from build123d import *

# Parameters (mm, degrees)
F0_W     = 26
F0_H     = 46
F1_DEPTH = 26
F2_W     = 10
F2_H     = 10
F3_DEPTH = 11
F4_W     = 10
F4_H     = 10
F5_DEPTH = 11
F7_R     = 1.55
F8_DEPTH = 26
F6_R     = 11
F9_DEPTH = 26


with BuildPart() as f1:
    # F0 (on Front) → F1 (new body)
    with BuildSketch(Plane.XZ):
        with Locations((13, 23)):
            Rectangle(F0_W, F0_H)
    extrude(amount=F1_DEPTH)

    # F2 (on face) → F3 (cut)
    with BuildSketch(Plane.XY.offset(46)):
        with Locations((13, -13)):
            Rectangle(F2_W, F2_H)
    extrude(amount=-F3_DEPTH, mode=Mode.SUBTRACT)

    # F4 (on face) → F5 (cut)
    with BuildSketch(Plane(origin=(0, 0, 0), x_dir=(1, 0, 0), z_dir=(0, 0, -1))):
        with Locations((13, 13)):
            Rectangle(F4_W, F4_H)
    extrude(amount=-F5_DEPTH, mode=Mode.SUBTRACT)

    # F7 (on face) → F8 (cut)
    with BuildSketch(Plane(origin=(0, 0, 0), x_dir=(0, -1, 0), z_dir=(-1, 0, 0))):
        with Locations((13, 8.5)):
            Circle(F7_R)
        with Locations((13, 3.5)):
            Circle(F7_R)
        with Locations((13, 42.5)):
            Circle(F7_R)
        with Locations((13, 37.5)):
            Circle(F7_R)
    extrude(amount=-F8_DEPTH, mode=Mode.SUBTRACT)

    # F6 (on face) → F9 (cut)
    with BuildSketch(Plane.YZ.offset(26)):
        with Locations((-13, 23)):
            Circle(F6_R)
    extrude(amount=-F9_DEPTH, mode=Mode.SUBTRACT)


solid = f1.part
Build history of the part. All positions in model axes, mm. A direction names the side the tool comes from. Give positions to 0.01 mm unless a question says otherwise; leave off trailing zeros. Order: outer loops, then holes, each group sorted by start corner. A loop starts at its lowest first (then second) coordinate and runs counter-clockwise, first axis right, second up. Notation, with made-up numbers: M 49,10.25 L 107,10.25 A20 cw 107,35.25 Z; hole C -35,58.25 d8. An arc over 180 degrees is marked long. Put each result on its own line as item: value.
Item 1: Slice it at D-D, the plane y = -7.5. Write the cut outline in (x, z), plus the area to 3 significant figures.
From the geometry:
outline: M 0,0 L 26,0 L 26,13.47 L 0,13.47 Z; M 0,32.53 L 26,32.53 L 26,46 L 0,46 Z
area: 701 mm2
Item 2: Two-plate mould, pull along Z, no slides. Class faces 4 (the cylindrical face through (13.18, -15.38, 12.26)), 5 (the cylindrical face through (3.944, -12.664, 40.987)), 6 (the flat face through (13, -13, 35)), 7 (the flat face through (8, -12.9, 5.4)): +Z half, -Z half, draft (parallel to the pull), parting line (faces both ways), or undercut.
From the geometry:
face 4: undercut
face 5: undercut
face 6: +Z half
face 7: draft
Item 3: Probe line 1 (Z direction, x = 3, y = -13); line 2 (X direction, y = -16.5, z = 10); line 3 (Z direction, x = 19.75, y = -20). List the from-to ranges inside material, lowest first. Write a range as [from, to].
From the geometry:
line 1: z = [0, 1.95], [5.05, 6.95], [10.05, 12], [34, 35.95], [39.05, 40.95], [44.05, 46]
line 2: x = [0, 8], [18, 26]
line 3: z = [0, 14.51], [31.49, 46]
Item 4: 3-axis set-ups, long thin cutter, end or side, ignore diameter. For faces 1 (the flat face through (8, -13.1, 40.6)), 2 (the flat face through (18, -12.9, 5.4)), 3 (the cylindrical face through (3.944, -12.664, 35.987)): which of +Z, -Z, +X, -X, +Y, -Y reach the whole face in a straight line?
From the geometry:
face 1: +Z
face 2: -Z
face 3: +X, -X
Item 5: Slice it at A-A, the plane z = 23. Write the cut outline in (x, y), plus the area to 3 significant figures.
From the geometry:
outline: M 0,-26 L 26,-26 L 26,-24 L 0,-24 Z; M 0,-2 L 26,-2 L 26,0 L 0,0 Z
area: 104 mm2
Item 6: Slice it at C-C, the plane x = 4. Write the cut outline in (y, z), plus the area to 3 significant figures.
From the geometry:
outline: M -26,0 L 0,0 L 0,46 L -26,46 Z; hole C -13,23 d22; hole C -13,3.5 d3.1; hole C -13,8.5 d3.1; hole C -13,37.5 d3.1; hole C -13,42.5 d3.1
area: 786 mm2
Item 7: Slice it at B-B, the plane x = 12. Write the cut outline in (y, z), plus the area to 3 significant figures.
From the geometry:
outline: M -26,0 L -18,0 L -18,11 L -8,11 L -8,0 L 0,0 L 0,46 L -8,46 L -8,35 L -18,35 L -18,46 L -26,46 Z; hole C -13,23 d22
area: 596 mm2
Item 8: Flat gauge pins, fed straight in: pin 1 Ø10 at (x, y) = (17, -20.5) entering from -Z; pin 2 Ø10 at (y, z) = (-12, 25) entering from +X. Where does each tip first touch, or does it go through?
From the geometry:
pin 1: stops at z = 0
pin 2: passes through
